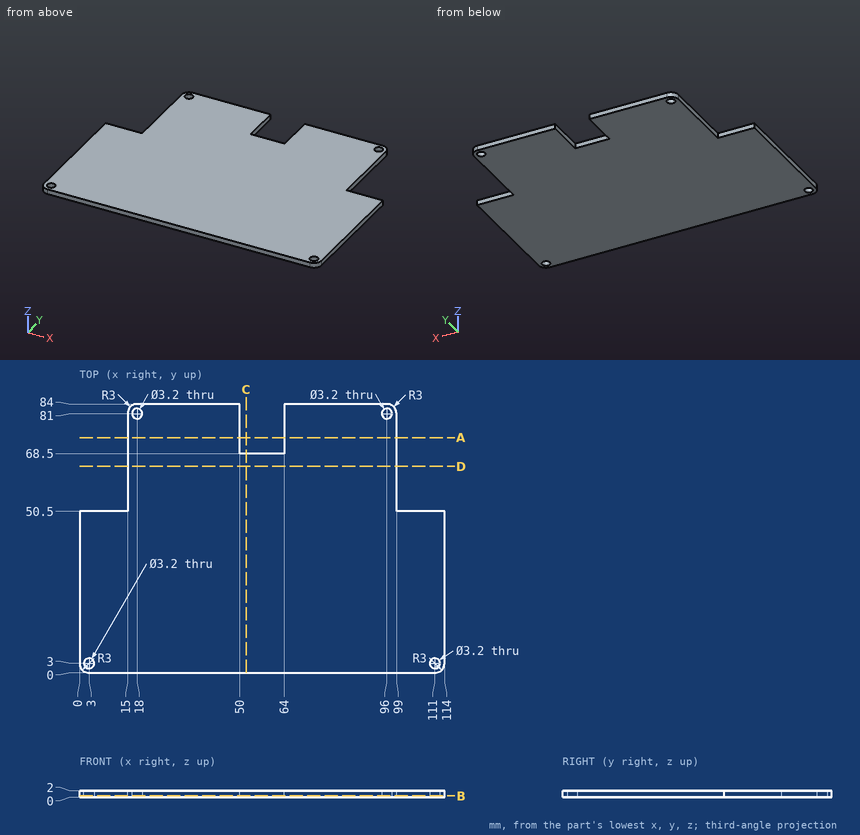
Verification items for this drawing (mm, ordinates from the low corner). Give positions to 0.01 mm unless a question says otherwise; leave off trailing zeros. Loops run counter-clockwise (first coordinate to the right, second up) from the corner with the lowest first, then second, coordinate; pieces in that order, holes last. Notation, with made-up numbers: (-0.5, 29.25) - (54.5, 29.25) arc R30 ccw to (54.5, 65.25) - close; hole circle Ø6 at (-10.5, 39.5). An arc over 180 degrees is marked (long way). Write item = value, one per line. Start each with the question number.
Q1. Cross-section at D-D, the plane y = 64.5. Enter the section's corners in (x, z).
Q2. Cross-section at A-A, the plane y = 73.5. Enter the section's corners in (x, z), and give its area (3 significant figures).
Q3. Cross-section at C-C, the plane x = 52. Enter the section's corners in (y, z), and give its area (3 significant figures).
Q4. Depth check by flat-ended pin: P1, Ø3, axis at x = 111, y = 3, coming from the +Z side; P2, Ø1, axis at x = 58, z = 0.5, coming from the +Y side; P3, Ø1, axis at y = 75.5, z = 1, coming from the +X side. Enter the tip coordinate at first touch or a pass-through.
Q5. Thickness scan on line 1 (X direction, y = 81, z = 1.5); line 2 (X direction, y = 71, z = 0.5); line 3 (Y direction, x = 111, z = 0.7). Record the ranges inside material, lowest first.
Q6. Cross-section at B-B, the plane z = 0.45. Enter the section's corners in (x, y).
Answer key:
q1.outline = (15, 0) - (99, 0) - (99, 2) - (15, 2) - close
q2.outline = (15, 0) - (50, 0) - (50, 2) - (15, 2) - close; (64, 0) - (99, 0) - (99, 2) - (64, 2) - close
q2.area = 140 mm^2
q3.outline = (0, 0) - (68.5, 0) - (68.5, 2) - (0, 2) - close
q3.area = 137 mm^2
q4.P1 = through
q4.P2 = 68.5
q4.P3 = 99
q5.line_1 = 15 to 16.4, 19.6 to 50, 64 to 94.4, 97.6 to 99
q5.line_2 = 15 to 50, 64 to 99
q5.line_3 = 0 to 1.4, 4.6 to 50.5
q6.outline = (0, 3) arc R3 ccw to (3, 0) - (111, 0) arc R3 ccw to (114, 3) - (114, 50.5) - (99, 50.5) - (99, 81) arc R3 ccw to (96, 84) - (64, 84) - (64, 68.5) - (50, 68.5) - (50, 84) - (18, 84) arc R3 ccw to (15, 81) - (15, 50.5) - (0, 50.5) - close; hole circle Ø3.2 at (3, 3); hole circle Ø3.2 at (18, 81); hole circle Ø3.2 at (96, 81); hole circle Ø3.2 at (111, 3)
